Work out the finished part from the listing and answer in its coordinate system (mm). Face numbers are marked on the shaded views. A direction names the side the tool comes from. Coordinates: 2 decimals unless noted, no trailing zeros. Write each loop counter-clockwise with the first axis right and the second up, starting at its lowest first coordinate (ties: lowest second). Pieces come first, ordered by that corner, then holes. Notation, with made-up numbers: (12, 55.25) - (38, 55.25) arc R18 cw to (38, 69.25) - close; hole circle Ø10 at (37, -15). An arc over 180 degrees is marked (long way). Use one line per item in the form item = value. Start each with the question number.
Item 1: Consider probe 1 along Y at (x, z) = (0, -3.8); probe 2 along Y at (x, z) = (0, -9); probe 3 along X at (y, z) = (-12, -5.25). Determine where each line is inside the solid, lowest interval first.
Item 2: Determine the mould class of the marked faces 3, 4 and 5 for opening direction Y: released by +Y, released by -Y, zero draft, split by the parting line, or undercut.
Item 3: Given pin 1 (12 mm diameter, centred on x = -8, z = -14.5, fed in from -Y); pin 2 (0.6 mm diameter, centred on x = -3, z = -15, fed in from -Y); pin 3 (7 mm diameter, centred on x = -20.57, y = -11.88, fed in from -Z), each flat-ended and moving along its own axis, determine where each tip first touches the part or whether it passes through.
Item 4: A cutting plane is placed at A-A (x = 0). Write down the section's boundary in (y, z), then the cut area to 3 significant figures.
Item 5: A cutting plane is placed at D-D (z = -23). Write down the section's boundary in (x, y), then the cut area to 3 significant figures.
Item 6: A cutting plane is placed at C-C (y = -7). Write down the section's boundary in (x, z), then the cut area to 3 significant figures.
Item 7: A cutting plane is placed at B-B (y = 1). Write down the section's boundary in (x, z), then the cut area to 3 significant figures.
Item 8: For the marked faces 1 and 2, determine the directions among +Z, -Z, +X, -X, +Y, -Y from which every point of the face is accessible in a straight line to the end or side of a thin tool.
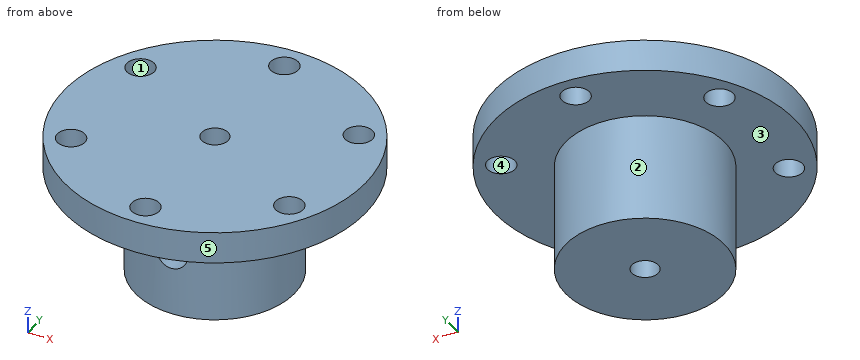
from build123d import *

# Parameters (mm, degrees)
SKETCH_2_R          = 2.5
CUT_EXTRUDE_1_DEPTH = 49.063291606
SKETCH_3_R          = 3
CUT_EXTRUDE_2_DEPTH = 49.063291606
SKETCH_4_R          = 2.6
CUT_EXTRUDE_3_DEPTH = 49.063291661


with BuildPart() as part:
    # 草图1 → 旋转1 (revolve)
    with BuildSketch(Plane(origin=(0, 0, 0), x_dir=(1, 0, 0), z_dir=(0, 1, 0))):
        Polygon((0, 0), (0, 26.4), (15, 26.4), (15, 6), (28.4, 6), (28.4, 0), align=None)
    revolve(axis=Axis((0, 0, 0), (0, 0, -1)))

    # 草图2 → 切除-拉伸1 (cut, through all)
    with BuildSketch(Plane(origin=(0, 0, -26.4), x_dir=(-1, 0, 0), z_dir=(0, 0, -1))):
        Circle(SKETCH_2_R)
    extrude(amount=-CUT_EXTRUDE_1_DEPTH, mode=Mode.SUBTRACT)

    # 草图3 → 切除-拉伸2 (cut, through all)
    with BuildSketch(Plane(origin=(0, 0, 0), x_dir=(1, 0, 0), z_dir=(0, 1, 0))):
        with Locations(Location((0, 14.370233869, 0), (0, 0, 270))):
            Circle(SKETCH_3_R)
    extrude(amount=-CUT_EXTRUDE_2_DEPTH, mode=Mode.SUBTRACT)

    # 草图4 → 切除-拉伸3 (cut, through all)
    with BuildSketch(Plane.XY):
        with Locations((0, 23.75)):
            Circle(SKETCH_4_R)
        with Locations((20.56810334, 11.875)):
            Circle(SKETCH_4_R)
        with Locations((20.56810334, -11.875)):
            Circle(SKETCH_4_R)
        with Locations((0, -23.75)):
            Circle(SKETCH_4_R)
        with Locations((-20.56810334, -11.875)):
            Circle(SKETCH_4_R)
        with Locations((-20.56810334, 11.875)):
            Circle(SKETCH_4_R)
    extrude(amount=-CUT_EXTRUDE_3_DEPTH, mode=Mode.SUBTRACT)


solid = part.part
Answer:
q1.probe_1 = -28.4 to -26.35, -21.15 to -2.5, 2.5 to 21.15, 26.35 to 28.4
q1.probe_2 = -15 to -2.5, 2.5 to 15
q1.probe_3 = -25.74 to -23.17, -17.97 to 17.97, 23.17 to 25.74
q2.face_3 = zero draft
q2.face_4 = undercut
q2.face_5 = split by the parting line
q3.pin_1 = -14.83
q3.pin_2 = -14.72
q3.pin_3 = -6
q4.outline = (-28.4, -6) - (-26.35, -6) - (-26.35, 0) - (-28.4, 0) - close; (-21.15, -6) - (-15, -6) - (-15, -11.37) - (-2.5, -11.37) - (-2.5, 0) - (-21.15, 0) - close; (-15, -26.4) - (-2.5, -26.4) - (-2.5, -17.37) - (-15, -17.37) - close; (2.5, -26.4) - (15, -26.4) - (15, -6) - (21.15, -6) - (21.15, 0) - (2.5, 0) - close; (26.35, -6) - (28.4, -6) - (28.4, 0) - (26.35, 0) - close
q4.area = 683 mm²
q5.outline = circle Ø30 at (0, 0); hole circle Ø5 at (0, 0)
q5.area = 687 mm²
q6.outline = (-27.52, -6) - (-13.27, -6) - (-13.27, -26.4) - (13.27, -26.4) - (13.27, -6) - (27.52, -6) - (27.52, 0) - (-27.52, 0) - close; hole circle Ø6 at (0, -14.37)
q6.area = 843 mm²
q7.outline = (-28.38, -6) - (-14.97, -6) - (-14.97, -26.4) - (-2.29, -26.4) - (-2.29, 0) - (-28.38, 0) - close; (2.29, -26.4) - (14.97, -26.4) - (14.97, -6) - (28.38, -6) - (28.38, 0) - (2.29, 0) - close
q7.area = 830 mm²
q8.face_1 = +Z, -Z
q8.face_2 = -Z
